Can you work these out from the model? Positions are in its coordinate system, mm. Face numbers are marked on the shaded views. Give positions to 0.01 mm unless a question says otherwise; leave off trailing zeros. Write each loop counter-clockwise with the first axis right and the second up, starting at its lowest first coordinate (ties: lowest second). Pieces come first, ordered by that corner, then holes.
1. Suppose I cut it at A-A (y = 48.5). Please give me the cut outline in (x, z) (3 decimals).
2. Suppose I cut it at B-B (y = 91.5). Give the number of separate pieces and of enclosed holes in the cut face, and give its area (3 significant figures).
3. If I drill on probe 1 along Y at (x, z) = (0, -2.45); probe 2 along Z at (x, y) = (-6, 81); probe 3 along X at (y, z) = (80.5, -10.25), over which ranges is the centre line in solid material (lowest first)?
4. I'm going to push flat-ended pins straight in: pin 1 (1.6 mm diameter, centred on x = 0, y = 78, fed in from +Z); pin 2 (0.8 mm diameter, centred on x = -4.5, z = 7.5, fed in from -Y); pin 3 (2 mm diameter, centred on x = 15.5, z = 1, fed in from -Y); pin 4 (1.5 mm diameter, centred on y = 92.5, z = -0.5, fed in from +X). Where does each tip first touch, or does it pass through?
5. Thinking about a two-plate mould opening in X: for the marked faces 1, 2, 3 and 4, which applies, pulls with the +X half, pulls with the -X half, needs draft (parallel to the pull), parting line crosses it, or undercut?
6. Suppose I cut it at C-C (x = 28). Please give me the cut outline in (y, z) (3 decimals).
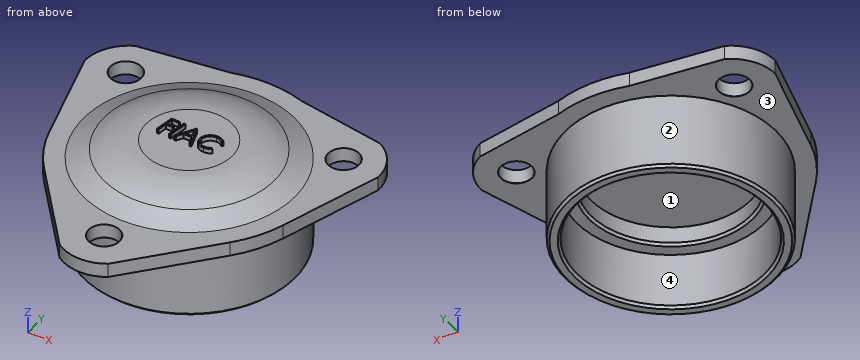
```python
from build123d import *

# Parameters (mm, degrees)
ESTRUSIONE_ESTRUSIONE2_DEPTH   = 3
RACCORDO1_R                    = 20
FORO_PER_VITE_M6_1_D           = 6.6
FORO_PER_VITE_M6_1_CSINK_D     = 6.65
FORO_PER_VITE_M6_1_CSINK_ANGLE = 90
ESTRUSIONE_ESTRUSIONE4_DEPTH   = 1
SCHIZZO13_R                    = 22.5
SCHIZZO13_R_2                  = 20
ESTRUSIONE_ESTRUSIONE5_DEPTH   = 16
SMUSSO1_SIZE                   = 0.5
SCHIZZO14_R                    = 20
SCHIZZO14_R_2                  = 17
ESTRUSIONE_ESTRUSIONE6_DEPTH   = 4
SMUSSO2_SIZE                   = 0.5


with BuildPart() as part:
    # Schizzo2 → Estrusione-Estrusione2 (new body)
    with BuildSketch(Plane.XY):
        with BuildLine():
            Line((31.811628146, 90.400572067), (25.390622586, 68.91275513))
            ThreePointArc((25.390622586, 68.91275513), (23.282129475, 63.843284505), (20.174211359, 59.317124919))
            Line((20.174211359, 59.317124919), (5.259333821, 41.805742776))
            ThreePointArc((5.259333821, 41.805742776), (0, 40.217089549), (-5.259333821, 41.805742776))
            Line((-5.259333821, 41.805742776), (-20.174211359, 59.317124919))
            ThreePointArc((-20.174211359, 59.317124919), (-23.282129475, 63.843284505), (-25.390622586, 68.91275513))
            Line((-25.390622586, 68.91275513), (-31.811628146, 90.400572067))
            ThreePointArc((-31.811628146, 90.400572067), (-30.431228874, 95.486838044), (-26.552294326, 99.054676397))
            Line((-26.552294326, 99.054676397), (-7.704995257, 101.855138495))
            ThreePointArc((-7.704995257, 101.855138495), (0, 103), (7.704995257, 101.855138495))
            Line((7.704995257, 101.855138495), (26.552294326, 99.054676397))
            ThreePointArc((26.552294326, 99.054676397), (30.431228874, 95.486838044), (31.811628146, 90.400572067))
        make_face()
    extrude(amount=ESTRUSIONE_ESTRUSIONE2_DEPTH)

    # Loft1: read off the stored shape, not the designer's step
    # Loft1: loft between two sections, ruled curve by curve
    loft1_from = [
        Edge.make_bspline([(-20.945888845, 84.717039643, 3), (-37.37996813, 42.825261952, 3), (4.51180956, 26.391182667, 3), (20.945888845, 68.282960357, 3), (37.37996813, 110.174738048, 3), (-4.51180956, 126.608817333, 3), (-20.945888845, 84.717039643, 3)], [0, 0, 0, 0, 0.5, 0.5, 0.5, 1, 1, 1, 1], 3, [1, 0.333333333, 0.333333333, 1, 0.333333333, 0.333333333, 1]),
    ]
    loft1_to = [
        Edge.make_bspline([(-8.243217943, 89.031933528, 7), (-33.307084999, 72.545497643, 7), (-16.820649113, 47.481630587, 7), (8.243217943, 63.968066472, 7), (33.307084999, 80.454502357, 7), (16.820649113, 105.518369413, 7), (-8.243217943, 89.031933528, 7)], [0, 0, 0, 0, 0.5, 0.5, 0.5, 1, 1, 1, 1], 3, [1, 0.333333333, 0.333333333, 1, 0.333333333, 0.333333333, 1]),
    ]
    loft1 = Solid(Shell([*[Face.make_surface_from_curves(loft1_from[k], loft1_to[k]) for k in range(1)], Face(Wire(loft1_from)), Face(Wire(loft1_to))]))
    add(loft1)

    # Raccordo1
    raccordo1_edges = [part.edges().sort_by_distance(p)[0] for p in [
        (8.243217943, 63.968066472, 7),
    ]]
    fillet(raccordo1_edges, radius=RACCORDO1_R)

    # Foro per Vite M6-1 (through all)
    with Locations(Plane(origin=(0, 0, 0), x_dir=(-1, 0, 0), z_dir=(0, 0, -1))):
        with Locations((-23.643180835, 91.5), (23.643180835, 91.5), (0, 48.5)):
            CounterSinkHole(FORO_PER_VITE_M6_1_D / 2, FORO_PER_VITE_M6_1_CSINK_D / 2, counter_sink_angle=FORO_PER_VITE_M6_1_CSINK_ANGLE)

    # Schizzo12 → Estrusione-Estrusione4 (add)
    # profile 1 of 4: a face of its own
    with BuildSketch(Plane.XY.offset(7)):
        Polygon((-3.596129901, 79), (-3.645008106, 78.641025641), (-5.13459144, 78.641025641), (-5.32209144, 77.307692308), (-3.852540158, 77.307692308), (-3.901418363, 76.948717949), (-5.371770927, 76.948717949), (-5.645008106, 75), (-6.006386312, 75), (-5.445488876, 79), align=None)
    # profile 2 of 4: a face of its own
    with BuildSketch(Plane.XY.offset(7)):
        Polygon((-2.778822209, 79), (-2.417444004, 79), (-2.97834144, 75), (-3.339719645, 75), align=None)
    # profile 3 of 4: a face of its own
    with BuildSketch(Plane.XY.offset(7)):
        Polygon((0.091370099, 79), (1.442331637, 75), (1.066530355, 75), (0.61540856, 76.333333333), (-1.145008106, 76.333333333), (-1.91984785, 75), (-2.326899132, 75), (-0.000777337, 79), align=None)
        Polygon((-0.032027337, 78.249198718), (-0.936674773, 76.692307692), (0.493613688, 76.692307692), align=None, mode=Mode.SUBTRACT)
    # profile 4 of 4: a face of its own
    with BuildSketch(Plane.XY.offset(7)):
        with BuildLine():
            Line((6.147459842, 78.461538462), (5.907075227, 78.128205128))
            add(Edge.make_bspline(
                [(5.907075227, 78.128205128), (5.853409068, 78.177252377), (5.748139309, 78.273461837), (5.57859512, 78.399066357), (5.403488099, 78.505445152), (5.22256522, 78.592311905), (5.036140145, 78.660469488), (4.844086397, 78.708187014), (4.646272643, 78.738264389), (4.512418126, 78.741801319), (4.444735483, 78.743589744)],
                knots=[0, 0, 0, 0, 1.071509858, 2.101838265, 3.105566767, 4.088534008, 5.056617788, 6.027134063, 7.002433514, 8, 8, 8, 8], degree=3))
            add(Edge.make_bspline(
                [(4.444735483, 78.743589744), (4.400373208, 78.742812621), (4.312286158, 78.741269543), (4.181334262, 78.729117344), (4.052913927, 78.708126456), (3.926602012, 78.679162503), (3.802411907, 78.64228048), (3.680155963, 78.597516258), (3.56054902, 78.543286131), (3.443628937, 78.482044458), (3.330601048, 78.414350152), (3.22428905, 78.33952652), (3.12333878, 78.259946704), (3.028834556, 78.174521349), (2.941380069, 78.082399604), (2.859264786, 77.98583622), (2.78482907, 77.882456135), (2.716015178, 77.774823109), (2.654558753, 77.663275365), (2.601448097, 77.548895655), (2.556421412, 77.432470171), (2.519611274, 77.31384374), (2.490613909, 77.193141896), (2.46962503, 77.070318011), (2.457497057, 76.945226207), (2.455936033, 76.861136633), (2.45515215, 76.818910256)],
                knots=[0, 0, 0, 0, 1.038808894, 2.06268977, 3.07662516, 4.084154014, 5.095481367, 6.108721937, 7.130613802, 8.168612606, 9.198437467, 10.213568377, 11.210969095, 12.207329739, 13.193903721, 14.183803377, 15.173465855, 16.174683957, 17.174102854, 18.153572289, 19.125845025, 20.09527659, 21.060177321, 22.030919679, 23.011207659, 24, 24, 24, 24], degree=3))
            add(Edge.make_bspline(
                [(2.45515215, 76.818910256), (2.455723998, 76.781491738), (2.456853287, 76.707597462), (2.467137224, 76.598513496), (2.481582904, 76.492331052), (2.504695805, 76.389786519), (2.532296075, 76.289652842), (2.567790414, 76.19322547), (2.608704098, 76.099685037), (2.655827766, 76.009788748), (2.709981947, 75.9244307), (2.767825544, 75.84203868), (2.833376205, 75.766228724), (2.903469648, 75.69420712), (2.979271851, 75.626878672), (3.06172917, 75.565604987), (3.148109174, 75.50693934), (3.241284048, 75.455918021), (3.337713946, 75.407825191), (3.439192633, 75.368472345), (3.543314355, 75.333536855), (3.651321135, 75.30582883), (3.762449094, 75.282865419), (3.877406714, 75.268399012), (3.995297146, 75.258117436), (4.075054043, 75.256983827), (4.11540856, 75.256410256)],
                knots=[0, 0, 0, 0, 1.050288761, 2.074115449, 3.074185512, 4.056755159, 5.022963132, 5.98847243, 6.938717655, 7.888015535, 8.834733031, 9.775342319, 10.711547043, 11.644864095, 12.595819208, 13.554196408, 14.527565762, 15.524707521, 16.534208059, 17.550758617, 18.577574426, 19.616152416, 20.679451723, 21.761233178, 22.867253411, 24, 24, 24, 24], degree=3))
            add(Edge.make_bspline(
                [(4.11540856, 75.256410256), (4.177436651, 75.257790942), (4.301068501, 75.260542869), (4.484631477, 75.282868048), (4.664978891, 75.318865819), (4.842002444, 75.369810901), (5.016050431, 75.43453316), (5.186569599, 75.514843771), (5.354579597, 75.607897574), (5.461316993, 75.681008093), (5.515248304, 75.717948718)],
                knots=[0, 0, 0, 0, 0.99335309, 1.979910703, 2.957437189, 3.936535413, 4.927536167, 5.928599034, 6.953381172, 8, 8, 8, 8], degree=3))
            Line((5.515248304, 75.717948718), (5.737203432, 75.401442308))
            add(Edge.make_bspline(
                [(5.737203432, 75.401442308), (5.698636022, 75.377400999), (5.623207082, 75.330381758), (5.510173423, 75.266138874), (5.402305276, 75.206488418), (5.298337121, 75.153355463), (5.198579513, 75.105882334), (5.1023715, 75.065337735), (5.011000051, 75.029494384), (4.892992217, 74.990590306), (4.74133145, 74.952952634), (4.550453852, 74.92005811), (4.346035685, 74.900897129), (4.205459903, 74.898612773), (4.133036765, 74.897435897)],
                knots=[0, 0, 0, 0, 0.95718736, 1.872037221, 2.738173064, 3.553405217, 4.331061281, 5.064628489, 5.752111019, 6.397930214, 7.680580555, 9.03930081, 10.474679465, 12, 12, 12, 12], degree=3))
            add(Edge.make_bspline(
                [(4.133036765, 74.897435897), (4.065668797, 74.898503504), (3.933826188, 74.900592864), (3.741149364, 74.921710204), (3.557866827, 74.95258651), (3.384436033, 74.999139462), (3.219772984, 75.056693596), (3.065642403, 75.129864143), (2.919625803, 75.213209751), (2.831076482, 75.280512719), (2.786882919, 75.314102564)],
                knots=[0, 0, 0, 0, 1.124936831, 2.201559726, 3.234383979, 4.226808245, 5.197736629, 6.143845973, 7.073622924, 8, 8, 8, 8], degree=3))
            add(Edge.make_bspline(
                [(2.786882919, 75.314102564), (2.758885291, 75.337621958), (2.703394402, 75.384237053), (2.62470229, 75.457997227), (2.551570012, 75.534983994), (2.484244847, 75.615533524), (2.42157733, 75.698321851), (2.365717698, 75.784759584), (2.313562827, 75.872994881), (2.268800829, 75.96512557), (2.22697839, 76.059317323), (2.192210864, 76.156942995), (2.16224319, 76.257459522), (2.138526146, 76.361127608), (2.119099109, 76.4674919), (2.105596966, 76.576905953), (2.097360113, 76.688973096), (2.09657437, 76.764675934), (2.096177791, 76.802884615)],
                knots=[0, 0, 0, 0, 1.031438255, 2.044295521, 3.04101972, 4.02510288, 5.004675323, 5.96814667, 6.927099159, 7.894246712, 8.855978008, 9.833229186, 10.815522105, 11.813498757, 12.831862773, 13.86462134, 14.922233219, 16, 16, 16, 16], degree=3))
            add(Edge.make_bspline(
                [(2.096177791, 76.802884615), (2.096577495, 76.842428296), (2.097372344, 76.921064649), (2.105650778, 77.037926676), (2.119089644, 77.152678707), (2.138604556, 77.264900109), (2.162372252, 77.374931575), (2.192108962, 77.482456198), (2.227496183, 77.587819052), (2.26846739, 77.690912174), (2.313946089, 77.792253604), (2.365597569, 77.890641468), (2.421437188, 77.987446425), (2.484309495, 78.080807656), (2.551867712, 78.172560242), (2.624363598, 78.262330978), (2.703619519, 78.348673131), (2.786172336, 78.433454544), (2.873429547, 78.514127778), (2.963688628, 78.590231175), (3.057030633, 78.660704389), (3.152310494, 78.726903249), (3.250787182, 78.786579776), (3.351531447, 78.841522422), (3.455054871, 78.891215855), (3.561207816, 78.935892226), (3.669937102, 78.975588021), (3.781394211, 79.008879856), (3.895516006, 79.0378999), (4.012061865, 79.061869924), (4.131310009, 79.08051087), (4.253292706, 79.092904794), (4.377840673, 79.101419939), (4.461815011, 79.102181335), (4.504030355, 79.102564103)],
                knots=[0, 0, 0, 0, 1.022044487, 2.032432208, 3.026697584, 4.007398125, 4.975698324, 5.935493653, 6.889610259, 7.847342231, 8.802158043, 9.759466851, 10.718641154, 11.689497925, 12.667180171, 13.663528933, 14.670419348, 15.695700261, 16.721678344, 17.740943913, 18.746223377, 19.744006424, 20.738655278, 21.721128384, 22.709310215, 23.705658978, 24.697235847, 25.699785021, 26.711210149, 27.740296491, 28.77439654, 29.829646392, 30.908925919, 32, 32, 32, 32], degree=3))
            add(Edge.make_bspline(
                [(4.504030355, 79.102564103), (4.580506116, 79.101020619), (4.730225931, 79.097998876), (4.949594324, 79.069889673), (5.158458449, 79.024831724), (5.324999268, 78.970585793), (5.454290614, 78.917658056), (5.552043217, 78.87243398), (5.649557753, 78.818839919), (5.748433722, 78.760454716), (5.84769365, 78.695580135), (5.947481515, 78.623682671), (6.04797544, 78.545625981), (6.1139998, 78.48982), (6.147459842, 78.461538462)],
                knots=[0, 0, 0, 0, 1.522680585, 2.981015879, 4.397098697, 5.773315249, 6.462902712, 7.179304435, 7.917249996, 8.678195189, 9.466166505, 10.278195975, 11.127418496, 12, 12, 12, 12], degree=3))
        make_face()
    extrude(amount=ESTRUSIONE_ESTRUSIONE4_DEPTH)

    # Schizzo13 → Estrusione-Estrusione5 (add)
    with BuildSketch(Plane(origin=(0, 0, 0), x_dir=(-1, 0, 0), z_dir=(0, 0, -1))):
        with Locations(Location((0, 76.5, 0), (0, 0, 180))):
            Circle(SCHIZZO13_R)
        with Locations((0, 76.5)):
            Circle(SCHIZZO13_R_2, mode=Mode.SUBTRACT)
    extrude(amount=ESTRUSIONE_ESTRUSIONE5_DEPTH)

    # Smusso1
    smusso1_edges = [part.edges().sort_by_distance(p)[0] for p in [
        (-22.5, 76.5, -16),
        (20, 76.5, -16),
    ]]
    chamfer(smusso1_edges, length=SMUSSO1_SIZE)

    # Schizzo14 → Estrusione-Estrusione6 (add)
    with BuildSketch(Plane(origin=(0, 0, 0), x_dir=(-1, 0, 0), z_dir=(0, 0, -1))):
        with Locations((0, 76.5)):
            Circle(SCHIZZO14_R)
        with Locations((0, 76.5)):
            Circle(SCHIZZO14_R_2, mode=Mode.SUBTRACT)
    extrude(amount=ESTRUSIONE_ESTRUSIONE6_DEPTH)

    # Smusso2
    smusso2_edges = [part.edges().sort_by_distance(p)[0] for p in [
        (17, 76.5, -4),
    ]]
    chamfer(smusso2_edges, length=SMUSSO2_SIZE)


solid = part.part
```
Checks:
1. outline: (-10.961, 0) - (-3.325, 0) - (-3.3, 0.025) - (-3.3, 3) - (-10.961, 3) - close; (3.3, 0.025) - (3.325, 0) - (10.961, 0) - (10.961, 3) - (3.3, 3) - close
2. separate pieces: 3
2. enclosed holes: 0
2. area: 373 mm2
3. probe 1: y = 54 to 59.5, 93.5 to 99
3. probe 2: z = 0 to 7
3. probe 3: x = -22.14 to -19.6, 19.6 to 22.14
4. pin 1: stops at z = 8
4. pin 2: stops at y = 76.95
4. pin 3: stops at y = 52.66
4. pin 4: stops at x = 31.71
5. face 1: undercut
5. face 2: parting line crosses it
5. face 3: needs draft
5. face 4: undercut
6. outline: (77.645, 0) - (98.163, 0) - (98.163, 3) - (77.645, 3) - close
